from build123d import *

# Parameters (mm, degrees)
SKETCH_1_R          = 20
SKETCH_1_R_2        = 2.05
EXTRUDE_1_DEPTH     = 7.5
SKETCH_2_R          = 1.25
SKETCH_2_R_2        = 12
CUT_EXTRUDE_1_DEPTH = 8.5
SKETCH_4_R          = 3.75
CUT_EXTRUDE_3_DEPTH = 5


with BuildPart() as part:
    # ｽｹｯﾁ1 → ﾎﾞｽ - 押し出し1 (new body)
    with BuildSketch(Plane.XY):
        Circle(SKETCH_1_R)
        with Locations((0, 15)):
            Circle(SKETCH_1_R_2, mode=Mode.SUBTRACT)
        with Locations((15, 0)):
            Circle(SKETCH_1_R_2, mode=Mode.SUBTRACT)
        with Locations((0, -15)):
            Circle(SKETCH_1_R_2, mode=Mode.SUBTRACT)
        with Locations((-15, 0)):
            Circle(SKETCH_1_R_2, mode=Mode.SUBTRACT)
    extrude(amount=EXTRUDE_1_DEPTH)

    # ｽｹｯﾁ2 → ｶｯﾄ - 押し出し1 (cut, through all)
    with BuildSketch(Plane.XY.offset(7.5)):
        with Locations((11.465736457, 11.465736457)):
            Circle(SKETCH_2_R)
        with Locations((-11.465736457, -11.465736457)):
            Circle(SKETCH_2_R)
        Circle(SKETCH_2_R_2)
    extrude(amount=-CUT_EXTRUDE_1_DEPTH, mode=Mode.SUBTRACT)

    # ｽｹｯﾁ4 → ｶｯﾄ - 押し出し3 (cut)
    with BuildSketch(Plane(origin=(0, 0, 0), x_dir=(-1, 0, 0), z_dir=(0, 0, -1))):
        with Locations((0, 15)):
            Circle(SKETCH_4_R)
        with Locations((15, 0)):
            Circle(SKETCH_4_R)
        with Locations((0, -15)):
            Circle(SKETCH_4_R)
        with Locations((-15, 0)):
            Circle(SKETCH_4_R)
    extrude(amount=-CUT_EXTRUDE_3_DEPTH, mode=Mode.SUBTRACT)


solid = part.part
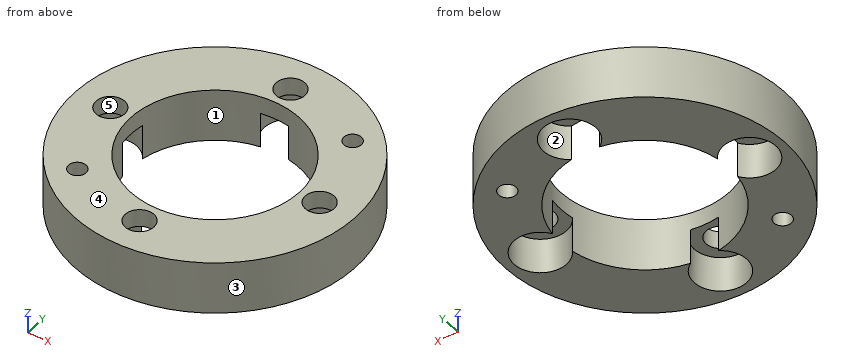
Geometry check sheet. Reference: the model listing, model coordinates, mm. Face numbers are marked on the shaded views. A direction names the side the tool comes from. Round coordinates to 2 decimals unless told otherwise and drop trailing zeros. Order: outer loops, then holes, each group sorted by start corner. A loop starts at its lowest first (then second) coordinate and runs counter-clockwise, first axis right, second up. Notation, with made-up numbers: (-31, 13) - (9, 13) arc R23 ccw to (9, 44) - close; hole circle Ø11 at (-23, 72). An arc over 180 degrees is marked (long way). One line per question, with ' | ' between items. Start each with the question number.
(1) Sectioned sample at D-D on z = 4.25. Record the cut outline in (x, y), and give its area (3 significant figures).
(2) Access from +Z, -Z, +X, -X, +Y, -Y to the whole of each face (thin tool, end or side, straight path). Record for the marked faces 1 and 2.
(3) Sectioned sample at C-C on y = -7.5. Record the cut outline in (x, z), and give its area (3 significant figures).
(4) Thickness scan on L1, parallel to Y at x = 0, z = 6; L2, parallel to X at y = -2.5, z = 3.75; L3, parallel to X at y = -11, z = 6.5. Record the ranges inside material, lowest first. Write a range as [from, to].
(5) Depth check by flat-ended pin: pin 1 Ø4.5 at (x, y) = (-15, 0) entering from +Z; pin 2 Ø4 at (x, z) = (-4, 6) entering from -Y; pin 3 Ø2 at (x, y) = (-1, -15.5) entering from -Z. Enter the tip coordinate at first touch or a pass-through.
(6) Release check for a two-part mould opening along X. For the marked faces 3, 4 and 5 record: released by +X, released by -X, zero draft, split by the parting line, or undercut.
(7) Sectioned sample at A-A on y = 0. Record the cut outline in (x, z), and give its area (3 significant figures).
Conclusion:
1) outline: circle Ø40 at (0, 0); hole circle Ø2.5 at (-11.47, -11.47); hole (-11.83, -2.01) arc R12 ccw to (-2.01, -11.83) arc R3.75 ccw (long way) to (2.01, -11.83) arc R12 ccw to (11.83, -2.01) arc R3.75 ccw (long way) to (11.83, 2.01) arc R12 ccw to (2.01, 11.83) arc R3.75 ccw (long way) to (-2.01, 11.83) arc R12 ccw to (-11.83, 2.01) arc R3.75 ccw (long way) to start; hole circle Ø2.5 at (11.47, 11.47) | area: 626 mm2
2) face 1: +Z, -Z | face 2: -Z
3) outline: (-18.54, 0) - (-9.37, 0) - (-9.37, 7.5) - (-18.54, 7.5) - close; (9.37, 0) - (18.54, 0) - (18.54, 7.5) - (9.37, 7.5) - close | area: 138 mm2
4) L1: y = [-20, -17.05], [-12.95, -12], [12, 12.95], [17.05, 20] | L2: x = [-19.84, -17.8], [-12.2, -11.74], [11.74, 12.2], [17.8, 19.84] | L3: x = [-16.7, -12.63], [-10.31, -4.8], [4.8, 16.7]
5) pin 1: stops at z = 7.5 | pin 2: stops at y = -19.9 | pin 3: stops at z = 5
6) face 3: split by the parting line | face 4: zero draft | face 5: undercut
7) outline: (-20, 0) - (-18.75, 0) - (-18.75, 5) - (-17.05, 5) - (-17.05, 7.5) - (-20, 7.5) - close; (-12.95, 5) - (-12, 5) - (-12, 7.5) - (-12.95, 7.5) - close; (12, 5) - (12.95, 5) - (12.95, 7.5) - (12, 7.5) - close; (17.05, 5) - (18.75, 5) - (18.75, 0) - (20, 0) - (20, 7.5) - (17.05, 7.5) - close | area: 32.0 mm2
